The model under review builds one solid part; all positions refer to its coordinate system, in mm. A direction names the side the tool comes from. Round coordinates to 2 decimals unless told otherwise and drop trailing zeros. Loops run counter-clockwise (first coordinate to the right, second up) from the corner with the lowest first, then second, coordinate; pieces in that order, holes last. Notation, with made-up numbers: M 36,-32 L 49,-32 A27 cw 49,-5 Z; hole C 7,46 d5. An arc over 180 degrees is marked long. Return JSON: item names as keys, results as strings. Group by question number.
Q1. Draft analysis for pull direction Y (two halves, no side actions). For faces 4 (the face through (38, 23.32, -101)), 5 (the face through (-28.89, 11.868, -107.045)), 6 (the face through (2, 4.762, -106)), state which applies: pulls with the +Y half, pulls with the -Y half, needs draft (parallel to the pull), parting line crosses it, or undercut.
Q2. To check wall thickness, follow line 1 along Z through (x, y) = (12.5, 23.5); line 2 along X through (y, z) = (18, -1) (3 decimals); line 3 along Z through (x, y) = (13.5, 9) (3 decimals). State the ranges of each line that lie inside material, in increasing order.
Q3. Consider section B-B (z = -48). State the section outline as (x, y) points (3 decimals).
Q4. Clearance check with flat-ended pins moving along their axes: pin 1 Ø10 at (y, z) = (17, -33.5) entering from -X (3 decimals); pin 2 Ø1.5 at (x, y) = (-12.5, 12) entering from -Z; pin 3 Ø7 at (x, z) = (36.195, 69.85) entering from -Y; pin 4 Ø2.5 at (x, z) = (-36.195, -101.6) entering from +Y. State where each tip first meets the part, or that it passes through.
Q5. For faces 1 (the face through (0, 9.525, -71)), 2 (the face through (-37, 23.32, 68)), 3 (the face through (20.32, 13, -107)), list the 3-axis set-ups (+Z, -Z, +X, -X, +Y, -Y) from which the entire face can be reached by the end or side of a thin tool; tool diameter is ignored.
from build123d import *

# Parameters (mm, degrees)
SKETCH1_W                                           = 59.69
SKETCH1_H                                           = 184.15
BOSS_EXTRUDE1_DEPTH                                 = 25.4
SHELL1_T                                            = -6.35
SKETCH2_W                                           = 46.99
SKETCH2_H                                           = 3.175
BOSS_EXTRUDE2_DEPTH                                 = 3.175
SKETCH3_W                                           = 12.7
SKETCH3_H                                           = 12.7
BOSS_EXTRUDE3_DEPTH                                 = 5.08
FILLET1_R                                           = 2.54
CBORE_FOR_00_BINDING_HEAD_MACHINE_SCREW_D           = 3.000000096
CBORE_FOR_00_BINDING_HEAD_MACHINE_SCREW_CBORE_D     = 5.999999938
CBORE_FOR_00_BINDING_HEAD_MACHINE_SCREW_CBORE_DEPTH = 3.000000096
SKETCH8_W                                           = 37.465
SKETCH8_H                                           = 15.875
CUT_EXTRUDE1_DEPTH                                  = 3.175
CUT_EXTRUDE2_REACH                                  = 189.636
SKETCH9_R                                           = 1.5
SKETCH9_W                                           = 32.7025
SKETCH9_H                                           = 12.7
FILLET2_R                                           = 1.5875
SKETCH10_W                                          = 4.7625
SKETCH10_H                                          = 4.7625
CUT_EXTRUDE3_DEPTH                                  = 4.7625
FILLET4_R                                           = 3.175


with BuildPart() as part:
    # Sketch1 → Boss-Extrude1 (new body)
    with BuildSketch(Plane(origin=(0, 0, 0), x_dir=(1, 0, 0), z_dir=(0, 1, 0))):
        with Locations((0, 15.875)):
            Rectangle(SKETCH1_W, SKETCH1_H)
    extrude(amount=BOSS_EXTRUDE1_DEPTH)

    # Shell1
    shell1_openings = [part.faces().sort_by_distance(p)[0] for p in [
        (0, 25.4, -15.875),
    ]]
    offset(amount=SHELL1_T, openings=shell1_openings, kind=Kind.INTERSECTION)

    # Sketch2 → Boss-Extrude2 (add)
    with BuildSketch(Plane(origin=(0, 6.35, 0), x_dir=(1, 0, 0), z_dir=(0, 1, 0))):
        with Locations((0, 71.4375)):
            Rectangle(SKETCH2_W, SKETCH2_H)
    extrude(amount=BOSS_EXTRUDE2_DEPTH)

    # Sketch3 → Boss-Extrude3 (add)
    with BuildSketch(Plane(origin=(0, 25.4, 0), x_dir=(1, 0, 0), z_dir=(0, 1, 0))):
        with Locations((-36.195, 101.6)):
            Rectangle(SKETCH3_W, SKETCH3_H)
        with Locations((-36.195, -69.85)):
            Rectangle(SKETCH3_W, SKETCH3_H)
        with Locations((36.195, -69.85)):
            Rectangle(SKETCH3_W, SKETCH3_H)
        with Locations((36.195, 101.6)):
            Rectangle(SKETCH3_W, SKETCH3_H)
    extrude(amount=-BOSS_EXTRUDE3_DEPTH)

    # Fillet1
    fillet1_edges = [part.edges().sort_by_distance(p)[0] for p in [
        (-29.845, 22.86, -95.25),
        (-42.545, 22.86, -95.25),
        (-42.545, 22.86, -107.95),
        (-29.845, 22.86, 63.5),
        (-42.545, 22.86, 76.2),
        (-42.545, 22.86, 63.5),
        (42.545, 22.86, 76.2),
        (29.845, 22.86, 63.5),
        (42.545, 22.86, 63.5),
        (42.545, 22.86, -107.95),
        (42.545, 22.86, -95.25),
        (29.845, 22.86, -95.25),
    ]]
    fillet(fillet1_edges, radius=FILLET1_R)

    # CBORE for #00 Binding Head Machine Screw1 (through all)
    with Locations(Plane(origin=(0, 20.32, 0), x_dir=(-1, 0, 0), z_dir=(0, -1, 0))):
        with Locations((-36.195, -69.85), (36.195, -69.85), (36.195, 101.6), (-36.195, 101.6)):
            CounterBoreHole(CBORE_FOR_00_BINDING_HEAD_MACHINE_SCREW_D / 2, CBORE_FOR_00_BINDING_HEAD_MACHINE_SCREW_CBORE_D / 2, CBORE_FOR_00_BINDING_HEAD_MACHINE_SCREW_CBORE_DEPTH)

    # Sketch8 → Cut-Extrude1 (cut)
    with BuildSketch(Plane(origin=(0, 0, -107.95), x_dir=(-1, 0, 0), z_dir=(0, 0, -1))):
        with BuildLine():
            ThreePointArc((17.145, 7.9375), (21.9075, 12.7), (17.145, 17.4625))
            Line((17.145, 17.4625), (17.145, 7.9375))
        make_face()
        with Locations((-1.5875, 12.7)):
            Rectangle(SKETCH8_W, SKETCH8_H)
    extrude(amount=-CUT_EXTRUDE1_DEPTH, mode=Mode.SUBTRACT)

    # Sketch9 → Cut-Extrude2 (cut, up to next)
    with BuildSketch(Plane(origin=(0, 0, -104.775), x_dir=(-1, 0, 0), z_dir=(0, 0, -1)), mode=Mode.PRIVATE) as cut_extrude2_sk1:
        with Locations((17.145, 12.7)):
            Circle(SKETCH9_R)
    cut_extrude2_tool1 = extrude(cut_extrude2_sk1.sketch, amount=-CUT_EXTRUDE2_REACH, mode=Mode.PRIVATE) & part.part
    # Sketch9 → Cut-Extrude2 (cut, up to next)
    with BuildSketch(Plane(origin=(0, 0, -104.775), x_dir=(-1, 0, 0), z_dir=(0, 0, -1)), mode=Mode.PRIVATE) as cut_extrude2_sk2:
        with Locations((-2.38125, 12.7)):
            Rectangle(SKETCH9_W, SKETCH9_H)
    cut_extrude2_tool2 = extrude(cut_extrude2_sk2.sketch, amount=-CUT_EXTRUDE2_REACH, mode=Mode.PRIVATE) & part.part
    add(cut_extrude2_tool1.solids().sort_by_distance((-17.145, 12.7, -104.775))[0], mode=Mode.SUBTRACT)
    add(cut_extrude2_tool2.solids().sort_by_distance((2.38125, 12.7, -104.775))[0], mode=Mode.SUBTRACT)

    # Fillet2
    fillet2_edges = [part.edges().sort_by_distance(p)[0] for p in [
        (-17.145, 4.7625, -106.3625),
        (20.32, 4.7625, -106.3625),
        (20.32, 20.6375, -106.3625),
        (-17.145, 20.6375, -106.3625),
        (18.7325, 19.05, -103.1875),
        (18.7325, 6.35, -103.1875),
        (-13.97, 6.35, -103.1875),
        (-13.97, 19.05, -103.1875),
    ]]
    fillet(fillet2_edges, radius=FILLET2_R)

    # Sketch10 → Cut-Extrude3 (cut)
    with BuildSketch(Plane.XY.offset(-101.6)):
        with Locations((21.11375, 12.7)):
            Rectangle(SKETCH10_W, SKETCH10_H)
    extrude(amount=-CUT_EXTRUDE3_DEPTH, mode=Mode.SUBTRACT)

    # Fillet4
    fillet4_edges = [part.edges().sort_by_distance(p)[0] for p in [
        (-29.845, 10.16, -107.95),
        (-29.845, 10.16, 76.2),
        (29.845, 0, -15.875),
        (0, 0, 76.2),
        (29.845, 10.16, 76.2),
        (-29.845, 0, -15.875),
        (0, 0, -107.95),
        (29.845, 10.16, -107.95),
    ]]
    fillet(fillet4_edges, radius=FILLET4_R)


solid = part.part
Values:
{
 "1": {"face 4": "pulls with the -Y half", "face 5": "needs draft", "face 6": "undercut"},
 "2": {"line 1": "z = -107.95 to -101.6, 69.85 to 76.2", "line 2": "x = -29.845 to -23.495, 23.495 to 29.845", "line 3": "z = -73.025 to -69.85, 69.85 to 76.2"},
 "3": {"outline": "M -29.845,3.175 A3.175 ccw -26.67,0 L 26.67,0 A3.175 ccw 29.845,3.175 L 29.845,25.4 L 23.495,25.4 L 23.495,6.35 L -23.495,6.35 L -23.495,25.4 L -29.845,25.4 Z"},
 "4": {"pin 1": "stops at x = -29.845", "pin 2": "stops at z = 69.85", "pin 3": "stops at y = 20.32", "pin 4": "passes through"},
 "5": {"face 1": "+Y", "face 2": "-Y", "face 3": "-Z"}
}
